CAD build for the part. Positions are in the model's coordinates, mm. Give positions to 0.01 mm unless a question says otherwise; leave off trailing zeros. Write each loop counter-clockwise with the first axis right and the second up, starting at its lowest first coordinate (ties: lowest second). Pieces come first, ordered by that corner, then holes. Notation, with made-up numbers: (86.25, 81) - (121.25, 81) arc R26 cw to (121.25, 120) - close; hole circle Ø7 at (41, 17.5). An arc over 180 degrees is marked (long way). Answer as a JSON object with one key per item and string values.
from build123d import *

# Parameters (mm, degrees)
F1_DEPTH = 2.5
F3_DEPTH = 25
F5_DEPTH = 25
F7_DEPTH = 25
F9_DEPTH = 2.5


with BuildPart() as f1:
    # F0 (on Top) → F1 (new body)
    with BuildSketch(Plane.XY):
        with BuildLine():
            ThreePointArc((155.8122909032, 0), (160.5434517066, 4.7311608034), (165.27461251, 0))
            Line((165.27461251, 0), (200, 0))
            Line((200, 0), (200, 6.6666666667))
            Line((200, 6.6666666667), (0, 9.6592448227))
            Line((0, 9.6592448227), (0, 0))
            Line((0, 0), (19.529893736, 0))
            ThreePointArc((19.529893736, 0), (25.529893736, 6), (31.529893736, 0))
            Line((31.529893736, 0), (59.1987557411, 0))
            ThreePointArc((59.1987557411, 0), (64.6987557411, 5.5), (70.1987557411, 0))
            Line((70.1987557411, 0), (102.6123418173, 0))
            ThreePointArc((102.6123418173, 0), (108.9262366295, 6.3138948122), (115.2401314417, 0))
            Line((115.2401314417, 0), (155.8122909032, 0))
        make_face()
        with BuildLine():
            Line((200, 0), (165.27461251, 0))
            ThreePointArc((165.27461251, 0), (160.5434517066, -4.7311608034), (155.8122909032, 0))
            Line((155.8122909032, 0), (115.2401314417, 0))
            ThreePointArc((115.2401314417, 0), (108.9262366295, -6.3138948122), (102.6123418173, 0))
            Line((102.6123418173, 0), (70.1987557411, 0))
            ThreePointArc((70.1987557411, 0), (64.6987557411, -5.5), (59.1987557411, 0))
            Line((59.1987557411, 0), (31.529893736, 0))
            ThreePointArc((31.529893736, 0), (25.529893736, -6), (19.529893736, 0))
            Line((19.529893736, 0), (0, 0))
            Line((0, 0), (0, -13.3407551773))
            Line((0, -13.3407551773), (200, -6.6666666667))
            Line((200, -6.6666666667), (200, 0))
        make_face()
    extrude(amount=F1_DEPTH)

    # F2 (on face) → F3 (cut)
    with BuildSketch(Plane.XY.offset(2.5)):
        Polygon((188.7384860036, 6.8351714706), (200, 0.3333333333), (200, 6.6666666667), align=None)
    extrude(amount=-F3_DEPTH, mode=Mode.SUBTRACT)

    # F4 (on face) → F5 (cut)
    with BuildSketch(Plane(origin=(0, 0, 0), x_dir=(1, 0, 0), z_dir=(0, 0, -1))):
        Polygon((195.8791541104, 6.8041811177), (200, -0.3333333333), (200, 6.6666666667), align=None)
    extrude(amount=-F5_DEPTH, mode=Mode.SUBTRACT)

    # F6 (on face) → F7 (cut)
    with BuildSketch(Plane(origin=(0, 0, 0), x_dir=(1, 0, 0), z_dir=(0, 0, -1))):
        Polygon((200, -0.3333333333), (199.3791541104, 0.7420032912), (186.1890294883, -6.87331871), (188.7384860036, -6.8351714706), align=None)
    extrude(amount=-F7_DEPTH, mode=Mode.SUBTRACT)

    # F8 (on face) → F9 (join)
    with BuildSketch(Plane(origin=(0, 0, 0), x_dir=(1, 0, 0), z_dir=(0, 0, -1))):
        Polygon((0, -9.6592448227), (0, 13.3407551773), (-23, 13.3407551773), align=None)
    extrude(amount=-F9_DEPTH)


solid = f1.part
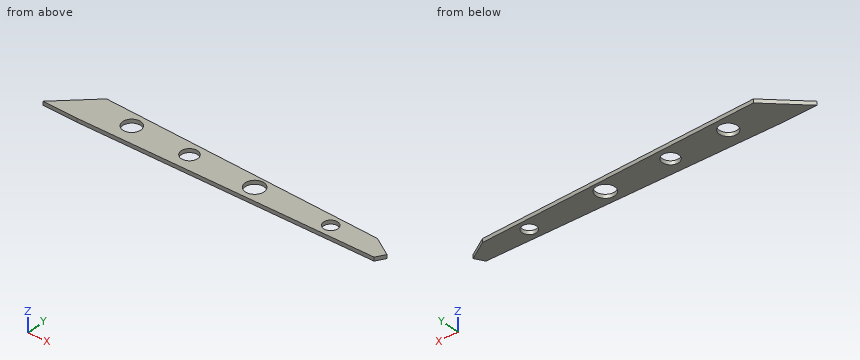
(1) Flat gauge pins, fed straight in: P1, Ø1.5, axis at y = 5.5, z = 1.5, coming from the -X side; P2, Ø10, axis at x = 64.7, y = 0, coming from the +Z side. Where does each tip first touch, or does it go through?
Answer key:
{"P1": "stops at x = -4.91", "P2": "passes through"}
(2) Saw through at A-A, the plane z = 1.35. Give the cut face in (x, y).
Answer key:
{"outline": "(-23, -13.34) - (0, -13.34) - (195.88, -6.8) - (199.38, -0.74) - (186.19, 6.87) - (0, 9.66) - close; hole circle Ø12 at (25.53, 0); hole circle Ø11 at (64.7, 0); hole circle Ø12.63 at (108.93, 0); hole circle Ø9.46 at (160.54, 0)"}
(3) Saw through at B-B, the plane x = 23.5. Give the cut face in (y, z), and give its area (3 significant figures).
Answer key:
{"outline": "(-12.56, 0) - (-5.65, 0) - (-5.65, 2.5) - (-12.56, 2.5) - close; (5.65, 0) - (9.31, 0) - (9.31, 2.5) - (5.65, 2.5) - close", "area": "26.4 mm²"}
(4) Saw through at C-C, the plane x = 170. Give the cut face in (y, z), and give its area (3 significant figures).
Answer key:
{"outline": "(-7.67, 0) - (7.12, 0) - (7.12, 2.5) - (-7.67, 2.5) - close", "area": "37.0 mm²"}
(5) Probe L1, parallel to X at y = 0.5, z = 1.1; L2, parallel to X at y = -3.75, z = 0.65; L3, parallel to X at y = 5, z = 1.8. List the from-to ranges inside material, lowest first. Write a range as [from, to].
Answer key:
{"L1": "x = [-9.16, 19.55], [31.51, 59.22], [70.18, 102.63], [115.22, 155.84], [165.25, 197.23]", "L2": "x = [-13.41, 20.85], [30.21, 60.68], [68.72, 103.85], [114.01, 157.66], [163.43, 197.64]", "L3": "x = [-4.66, 22.21], [28.85, 62.41], [66.99, 105.07], [112.78, 189.43]"}
